Verification items for the finished model (mm, model axes). A direction names the side the tool comes from. Coordinates: 2 decimals unless noted, no trailing zeros. Write each loop counter-clockwise with the first axis right and the second up, starting at its lowest first coordinate (ties: lowest second). Pieces come first, ordered by that corner, then holes. Notation, with made-up numbers: (-1, -9.75) -> (46, -9.75) arc R16 ccw to (46, 19.25) -> close; hole circle Ø7 at (70, 52). An arc over 180 degrees is marked (long way). Write item = value, one per line. Start each with the question number.
(1) Mould release check, pull along Y, two halves, no side actions. Record for faces 4 (the face through (-19.24, 45.57, 9.06)), 5 (the face through (-12, 27, 0)), 6 (the face through (-12, 0, 29)): released by +Y, released by -Y, zero draft, split by the parting line, or undercut.
(2) Set-up check for faces 1 (the face through (-10.83, 46.96, 46.69)), 2 (the face through (-24, 27.2, 28.6)), 3 (the face through (-1, 37, 29)): record each of +Z, -Z, +X, -X, +Y, -Y from which the full face is reachable in a straight line by a thin tool's end or side.
(3) Section check B-B (x = -1.5). Record the cut outline in (y, z).
(4) Gauge pin test, flat ends, axial feed: pin 1 Ø8.5 at (y, z) = (49.5, 29) entering from +X; pin 2 Ø8.5 at (y, z) = (20, 29) entering from +X (3 decimals); pin 3 Ø4 at (y, z) = (46, 9) entering from +X; pin 4 Ø2.5 at (x, z) = (-1, 27) entering from +Y. Record the tip position at first contact, or that the pin passes through.
(5) Section check A-A (z = 29). Record the cut outline in (x, y).
(6) Section check D-D (x = -12.75). Record the cut outline in (y, z).
(7) Material ranges on probe 1 along Y at (x, z) = (-11.5, 9); probe 2 along Z at (x, y) = (-22.25, 22.5); probe 3 along X at (y, z) = (41.5, 16.5), recorded low to high. Write a range as [from, to].
(8) Section check C-C (y = 20). Record the cut outline in (x, z).
```python
from build123d import *

# Parameters (mm, degrees)
BOSS_EXTRU_1_DEPTH         = 58
ESQUISSE2_R                = 5
ENL_V_MAT_EXTRU_1_DEPTH    = 83.800966178
TROU_TARAUD_M161_D         = 14
R_P_TITION_LIN_AIRE1_COUNT = 2
R_P_TITION_LIN_AIRE1_PITCH = 40


with BuildPart() as part:
    # Esquisse1 → Boss.-Extru.1 (new body)
    with BuildSketch(Plane.XY):
        Polygon((0, 0), (0, 37), (-3, 37), (-3, 54), (-14, 54), (-24, 44), (-24, 0), align=None)
    extrude(amount=BOSS_EXTRU_1_DEPTH)

    # Esquisse2 → Enlèv. mat.-Extru.1 (cut, through all)
    with BuildSketch(Plane(origin=(0, 0, 0), x_dir=(0, 0, -1), z_dir=(1, 0, 0))):
        with Locations((-9, 20)):
            Circle(ESQUISSE2_R)
        with Locations(Location((-49, 20, 0), (0, 0, 180))):
            Circle(ESQUISSE2_R)
    extrude(amount=-ENL_V_MAT_EXTRU_1_DEPTH, mode=Mode.SUBTRACT)

    # Trou taraudé M161 (through all)
    with Locations(Plane(origin=(0, 0, 0), x_dir=(0, 0, -1), z_dir=(1, 0, 0))):
        with Locations((-29, 20)):
            Hole(TROU_TARAUD_M161_D / 2)

    # Esquisse8 → Trou taraudé M61 (revolve, cut)
    with BuildSketch(Plane(origin=(-3, 46, 9), x_dir=(0, 0, -1), z_dir=(0, 1, 0))):
        Polygon((0, 0), (0, 16.502151548), (2.5, 15), (2.5, 0.866025404), (4, 0), align=None)
    trou_taraud_m61 = revolve(axis=Axis((3.35, 46, 9), (-1, 0, 0)), mode=Mode.SUBTRACT)

    # Répétition linéaire1: Trou taraudé M61 ×2
    with Locations(*[(0, 0, i * R_P_TITION_LIN_AIRE1_PITCH) for i in range(1, R_P_TITION_LIN_AIRE1_COUNT)]):
        add(trou_taraud_m61, mode=Mode.SUBTRACT)


solid = part.part
```
Response:
q1.face_4 = undercut
q1.face_5 = zero draft
q1.face_6 = released by -Y
q2.face_1 = +X
q2.face_2 = +Z, -Z, -X, +Y, -Y
q2.face_3 = +Z, -Z, +X, +Y
q3.outline = (0, 0) -> (37, 0) -> (37, 58) -> (0, 58) -> close; hole circle Ø14 at (20, 29); hole circle Ø10 at (20, 9); hole circle Ø10 at (20, 49)
q4.pin_1 = -3
q4.pin_2 = through
q4.pin_3 = -18.3
q4.pin_4 = 37
q5.outline = (-24, 0) -> (0, 0) -> (0, 13) -> (-24, 13) -> close; (-24, 27) -> (0, 27) -> (0, 37) -> (-3, 37) -> (-3, 54) -> (-14, 54) -> (-24, 44) -> close
q6.outline = (0, 0) -> (54, 0) -> (54, 58) -> (0, 58) -> close; hole circle Ø14 at (20, 29); hole circle Ø10 at (20, 9); hole circle Ø10 at (20, 49); hole circle Ø5 at (46, 9); hole circle Ø5 at (46, 49)
q7.probe_1 = [0, 15], [25, 43.5], [48.5, 54]
q7.probe_2 = [0, 4.67], [13.33, 22.46], [35.54, 44.67], [53.33, 58]
q7.probe_3 = [-24, -3]
q8.outline = (-24, 0) -> (0, 0) -> (0, 4) -> (-24, 4) -> close; (-24, 14) -> (0, 14) -> (0, 22) -> (-24, 22) -> close; (-24, 36) -> (0, 36) -> (0, 44) -> (-24, 44) -> close; (-24, 54) -> (0, 54) -> (0, 58) -> (-24, 58) -> close
